Here's how the part is built. I have some questions about the finished solid (model axes, mm). A direction names the side the tool comes from. Coordinates: 2 decimals unless noted, no trailing zeros. Write each loop counter-clockwise with the first axis right and the second up, starting at its lowest first coordinate (ties: lowest second). Pieces come first, ordered by that corner, then holes.
from build123d import *

# Parameters (mm, degrees)
SKETCH1_R           = 1.125
BOSS_EXTRUDE1_DEPTH = 5
CUT_EXTRUDE1_START  = -2
SKETCH2_R           = 1.125
CUT_EXTRUDE1_DEPTH  = 2
SKETCH3_R           = 1.125
CUT_EXTRUDE2_DEPTH  = 1.5
CUT_EXTRUDE3_DEPTH  = 2


with BuildPart() as part:
    # Sketch1 → Boss-Extrude1 (new body)
    with BuildSketch(Plane(origin=(0, 0, 0), x_dir=(1, 0, 0), z_dir=(0, 1, 0))):
        with BuildLine():
            ThreePointArc((-4.248671667, 0.10625), (0, -4.25), (4.248671667, 0.10625))
            Line((4.248671667, 0.10625), (3.748827942, 20.09375))
            ThreePointArc((3.748827942, 20.09375), (0, 23.75), (-3.748827942, 20.09375))
            Line((-3.748827942, 20.09375), (-4.248671667, 0.10625))
        make_face()
        with Locations(Location((0, 0, 0), (0, 0, 270))):
            Circle(SKETCH1_R, mode=Mode.SUBTRACT)
        with Locations(Location((0, 20, 0), (0, 0, 270))):
            Circle(SKETCH1_R, mode=Mode.SUBTRACT)
    extrude(amount=BOSS_EXTRUDE1_DEPTH)

    # Sketch2 → Cut-Extrude1 (cut)
    # profile 1 of 2: a face of its own
    with BuildSketch(Plane(origin=(0, 5, 0), x_dir=(1, 0, 0), z_dir=(0, 1, 0)).offset(CUT_EXTRUDE1_START)):
        with BuildLine():
            ThreePointArc((2.225, 1.780975856), (-2.689214569, -0.943729304), (2.85, 0))
            ThreePointArc((2.85, 0), (2.689214569, 0.943729304), (2.225, 1.780975856))
        make_face()
        with Locations(Location((0, 0, 0), (0, 0, 270))):
            Circle(SKETCH2_R, mode=Mode.SUBTRACT)
    # profile 2 of 2: a face of its own
    with BuildSketch(Plane(origin=(0, 5, 0), x_dir=(1, 0, 0), z_dir=(0, 1, 0)).offset(CUT_EXTRUDE1_START)):
        with BuildLine():
            ThreePointArc((2.225, 1.780975856), (2.689214569, 0.943729304), (2.85, 0))
            Line((2.85, 0), (2.85, 15))
            Line((2.85, 15), (2.225, 15))
            Line((2.225, 15), (2.225, 1.780975856))
        make_face()
    extrude(amount=CUT_EXTRUDE1_DEPTH, mode=Mode.SUBTRACT)

    # Sketch3 → Cut-Extrude2 (cut)
    with BuildSketch(Plane.XZ):
        Polygon((2.125, -1.226869322), (2.125, 1.226869322), (0, 2.453738644), (-2.125, 1.226869322), (-2.125, -1.226869322), (0, -2.453738644), align=None)
        with Locations(Location((0, 0, 0), (0, 0, 270))):
            Circle(SKETCH3_R, mode=Mode.SUBTRACT)
    extrude(amount=-CUT_EXTRUDE2_DEPTH, mode=Mode.SUBTRACT)

    # Sketch3_3 → Cut-Extrude3 (cut)
    with BuildSketch(Plane.XZ):
        Polygon((2.125, -21.226869322), (0, -22.453738644), (-2.125, -21.226869322), (-2.125, -18.773130678), (0, -17.546261356), (2.125, -18.773130678), align=None)
    extrude(amount=-CUT_EXTRUDE3_DEPTH, mode=Mode.SUBTRACT)


solid = part.part
1. For pin 1 Ø1 at (y, z) = (1.5, -9) entering from -X; pin 2 Ø0.6 at (y, z) = (4, -10.5) entering from +X; pin 3 Ø1 at (y, z) = (0.5, -19.5) entering from +X; pin 4 Ø3.5 at (x, z) = (-1, -1) entering from -Y, each with a flat end and sliding along its axis, tell me the tip position at first contact or that it passes through.
2. If I drill on line 1 (Z direction, x = 0, y = 3.9) (3 decimals); line 2 (X direction, y = 2.75, z = -20) (3 decimals); line 3 (X direction, y = 1.9, z = 0) (3 decimals), over which ranges is the centre line in solid material (lowest first)?
3. I want a section at D-D (x = 1.5). List the corners of the cut face in (y, z) for me.
4. I want a section at C-C (z = -17). List the corners of the cut face in (x, y) for me, then the cut area to 3 significant figures.
5. I want a section at A-A (y = 3.75). List the corners of the cut face in (x, z) for me (3 decimals), then the cut area to 3 significant figures.
6. On a 3-axis mill with a long thin cutter (end or side, diameter ignored), from which of +Z, -Z, +X, -X, +Y, -Y can I reach the whole of each face in a straight line? I mean faces 1 (the face through (0.338, 2.24, 1.073)), 2 (the face through (-1.08, 0.74, -1.83)), 3 (the face through (2.225, 4, -8)). Say none if no direction works.
7. I want a section at B-B (x = -1.75). List the corners of the cut face in (y, z) for me.
Response values:
1. pin 1: stops at x = -4.04
1. pin 2: stops at x = 4
1. pin 3: stops at x = 3.78
1. pin 4: stops at y = 0
2. line 1: z = -23.75 to -21.125, -18.875 to -2.85, 2.85 to 4.25
2. line 2: x = -3.751 to -1.125, 1.125 to 3.751
2. line 3: x = -4.25 to -1.125, 1.125 to 4.25
3. outline: (0, -23.44) - (5, -23.44) - (5, -2.42) - (3, -2.42) - (3, 2.42) - (5, 2.42) - (5, 3.98) - (0, 3.98) - (0, 1.59) - (1.5, 1.59) - (1.5, -1.59) - (0, -1.59) - (0, -18.41) - (2, -18.41) - (2, -21.59) - (0, -21.59) - close
4. outline: (-3.83, 0) - (3.83, 0) - (3.83, 5) - (-3.83, 5) - close
4. area: 38.3 mm2
5. outline: (-4.249, -0.106) - (-3.749, -20.094) arc R3.75 ccw to (3.749, -20.094) - (4.249, -0.106) arc R4.25 ccw (long way) to start; hole circle Ø2.25 at (0, -20); hole (2.225, -15) - (2.85, -15) - (2.85, 0) arc R2.85 ccw (long way) to (2.225, -1.781) - close
5. area: 172 mm2
6. face 1: +Y, -Y
6. face 2: -Y
6. face 3: +Y
7. outline: (0, -23.32) - (5, -23.32) - (5, -2.25) - (3, -2.25) - (3, 2.25) - (5, 2.25) - (5, 3.87) - (0, 3.87) - (0, 1.44) - (1.5, 1.44) - (1.5, -1.44) - (0, -1.44) - (0, -18.56) - (2, -18.56) - (2, -21.44) - (0, -21.44) - close
